Here's the drawing with two shaded views (mm, measured from the low corner). I have some questions. Round coordinates to 2 decimals unless told otherwise and drop trailing zeros. Loops run counter-clockwise (first coordinate to the right, second up) from the corner with the lowest first, then second, coordinate; pieces in that order, holes last. Notation, with made-up numbers: (19.25, -30) -> (28.25, -30) arc R12 ccw to (28.25, -18) -> close; hole circle Ø6 at (10, 11.5). An arc over 180 degrees is marked (long way). Use a Markdown table: item, result.
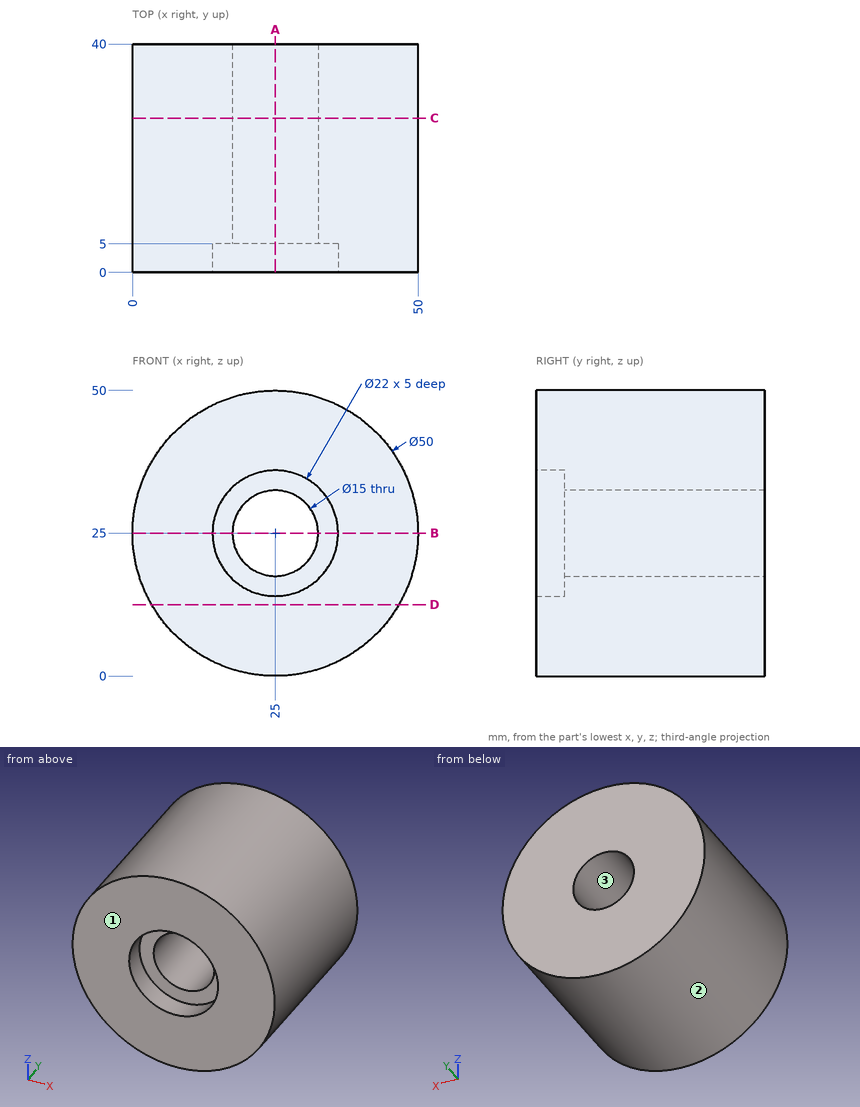
1. Will these pins go through, and if not, where does the flat tip stop? pin 1 Ø1 at (x, z) = (31, 5.5) entering from -Y; pin 2 Ø2 at (x, y) = (6.5, 32) entering from +Z; pin 3 Ø1 at (x, y) = (16, 28) entering from -Z; pin 4 Ø6.5 at (x, z) = (25.5, 28) entering from -Y.
Answer sheet:
| item | result |
|---|---|
| pin 1 | stops at y = 0 |
| pin 2 | stops at z = 42.85 |
| pin 3 | stops at z = 1.49 |
| pin 4 | passes through |
2. I want a section at D-D (z = 12.5). Please give me the cut outline in (x, y), plus the area to 3 significant figures.
Answer sheet:
| item | result |
|---|---|
| outline | (3.35, 0) -> (46.65, 0) -> (46.65, 40) -> (3.35, 40) -> close |
| area | 1,730 mm² |
3. I want a section at B-B (z = 25). Please give me the cut outline in (x, y).
Answer sheet:
| item | result |
|---|---|
| outline | (0, 0) -> (14, 0) -> (14, 5) -> (17.5, 5) -> (17.5, 40) -> (0, 40) -> close; (32.5, 5) -> (36, 5) -> (36, 0) -> (50, 0) -> (50, 40) -> (32.5, 40) -> close |
4. I want a section at C-C (y = 27). Please give me the cut outline in (x, z), plus the area to 3 significant figures.
Answer sheet:
| item | result |
|---|---|
| outline | circle Ø50 at (25, 25); hole circle Ø15 at (25, 25) |
| area | 1,790 mm² |
5. I want a section at A-A (x = 25). Please give me the cut outline in (y, z), plus the area to 4 significant figures.
Answer sheet:
| item | result |
|---|---|
| outline | (0, 0) -> (40, 0) -> (40, 17.5) -> (5, 17.5) -> (5, 14) -> (0, 14) -> close; (0, 36) -> (5, 36) -> (5, 32.5) -> (40, 32.5) -> (40, 50) -> (0, 50) -> close |
| area | 1,365 mm² |
6. I need wall thicknesses on line 1 (X direction, y = 17, z = 25); line 2 (X direction, y = 1.35, z = 25); line 3 (Z direction, x = 19.5, y = 12). Which ranges of each line are inside material? Lowest first, please.
Answer sheet:
| item | result |
|---|---|
| line 1 | x = 0 to 17.5, 32.5 to 50 |
| line 2 | x = 0 to 14, 36 to 50 |
| line 3 | z = 0.61 to 19.9, 30.1 to 49.39 |
7. If we mould it in two halves opening along X, with no side actions, what happens to the marked faces 1, 2 and 3? For each: +X half, -X half, draft (parallel to the pull), parting line (faces both ways), or undercut.
Answer sheet:
| item | result |
|---|---|
| face 1 | draft |
| face 2 | parting line |
| face 3 | undercut |
